Design review of the part built by this model. Coordinates are the model's own, in mm. A direction names the side the tool comes from. Give positions to 0.01 mm unless a question says otherwise; leave off trailing zeros. Write each loop counter-clockwise with the first axis right and the second up, starting at its lowest first coordinate (ties: lowest second). Pieces come first, ordered by that corner, then holes. Notation, with made-up numbers: M 10.25,-21.75 L 15.25,-21.75 A17 cw 15.25,5.25 Z; hole C 23.25,48 d1. An arc over 180 degrees is marked long. Use a Markdown table: item, result. Add a question column.
```python
from build123d import *

# Parameters (mm, degrees)
SKETCH2_R           = 2
BOSS_EXTRUDE1_DEPTH = 2.5


with BuildPart() as part:
    # Sketch2 → Boss-Extrude1 (new body)
    with BuildSketch(Plane.XY):
        with BuildLine():
            Line((-8.825, 5.0000164), (8.825, 5.0000164))
            ThreePointArc((8.825, 5.0000164), (12.499924895, -2.3221e-05), (8.825, -5.000062843))
            Line((8.825, -5.000062843), (-8.825, -5.000062843))
            ThreePointArc((-8.825, -5.000062843), (-12.499924895, -2.3221e-05), (-8.825, 5.0000164))
        make_face()
        with Locations((-8.825, -2.3221e-05)):
            Circle(SKETCH2_R, mode=Mode.SUBTRACT)
        with Locations(Location((8.825, -2.3221e-05, 0), (0, 0, 180))):
            Circle(SKETCH2_R, mode=Mode.SUBTRACT)
        Polygon((-5.125, -2.725), (-5.125, 2.725), (-5.125, 3.625), (-3.085, 3.625), (3.085, 3.625), (5.125, 3.625), (5.125, 2.725), (5.125, -2.725), (5.125, -3.625), (3.085, -3.625), (-3.085, -3.625), (-5.125, -3.625), align=None, mode=Mode.SUBTRACT)
    extrude(amount=BOSS_EXTRUDE1_DEPTH)


solid = part.part
```
(1) For pin 1 (1.2 mm diameter, centred on y = -1, z = 1.5, fed in from +X); pin 2 (1.2 mm diameter, centred on y = 1.5, z = 1, fed in from -X), all flat-tipped, find the tip position at first contact; note any pin that passes through.
(2) Machinability: for faces 1 (the cylindrical face through (-12.5, -0.1, 1.2)), 2 (the flat face through (5.125, 0, 1)), which of the approach directions +Z, -Z, +X, -X, +Y, -Y give a long, thin tool a straight path to every point of the face, cutting with its end or side? Answer none if there is none.
(3) The part is to be moulded in two halves that separate along Y. For faces 3 (the flat face through (0, 5, 1)), 4 (the cylindrical face through (-6.98, -0.77, 1.23)), 5 (the flat face through (0, -5, 1)), say which applies: released by +Y, released by -Y, zero draft, split by the parting line, or undercut.
(4) Add section C-C on z = 0.95. Give the boundary of the cut face in (x, y) (3 decimals).
(5) Add section D-D on y = 3. Give the boundary of the cut face in (x, z) (3 decimals), then the cut area to 3 significant figures.
(6) Wall thickness on L1, parallel to Y at x = -4, z = 2 (3 decimals); L2, parallel to X at y = -1.25, z = 1.8 (3 decimals); L3, parallel to X at y = -0.5, z = 1.1 (1 decimal): over which ranges is each line inside the solid? List them lowest first.
(7) Add section B-B on y = -1.5. Give the boundary of the cut face in (x, z) (3 decimals).
(8) Add section A-A on x = 0.5. Give the boundary of the cut face in (y, z) (3 decimals), then the cut area to 3 significant figures.
From the geometry:
| question | item | result |
|---|---|---|
| 1 | pin 1 | stops at x = 12.48 |
| 1 | pin 2 | stops at x = -12.42 |
| 2 | face 1 | +Z, -Z, -X |
| 2 | face 2 | +Z, -Z |
| 3 | face 3 | released by +Y |
| 3 | face 4 | undercut |
| 3 | face 5 | released by -Y |
| 4 | outline | M -8.825,-5 L 8.825,-5 A5.239 ccw 8.825,5 L -8.825,5 A5.239 ccw Z; hole C -8.825,0 d4; hole M -5.125,-3.625 L 5.125,-3.625 L 5.125,3.625 L -5.125,3.625 Z; hole C 8.825,0 d4 |
| 5 | outline | M -11.556,0 L -5.125,0 L -5.125,2.5 L -11.556,2.5 Z; M 5.125,0 L 11.556,0 L 11.556,2.5 L 5.125,2.5 Z |
| 5 | area | 32.2 mm^2 |
| 6 | L1 | y = -5 to -3.625, 3.625 to 5 |
| 6 | L2 | x = -12.349 to -10.386, -7.264 to -5.125, 5.125 to 7.264, 10.386 to 12.349 |
| 6 | L3 | x = -12.5 to -10.8, -6.9 to -5.1, 5.1 to 6.9, 10.8 to 12.5 |
| 7 | outline | M -12.281,0 L -10.148,0 L -10.148,2.5 L -12.281,2.5 Z; M -7.502,0 L -5.125,0 L -5.125,2.5 L -7.502,2.5 Z; M 5.125,0 L 7.502,0 L 7.502,2.5 L 5.125,2.5 Z; M 10.148,0 L 12.281,0 L 12.281,2.5 L 10.148,2.5 Z |
| 8 | outline | M -5,0 L -3.625,0 L -3.625,2.5 L -5,2.5 Z; M 3.625,0 L 5,0 L 5,2.5 L 3.625,2.5 Z |
| 8 | area | 6.88 mm^2 |
